from build123d import *

# Parameters (mm, degrees)
SKETCH2_R           = 49.2125
BOSS_EXTRUDE1_DEPTH = 50.8
SKETCH3_R           = 9.525
SKETCH4_R           = 49.2125
SKETCH4_R_2         = 9.525
BOSS_EXTRUDE2_DEPTH = 50.8


with BuildPart() as part:
    # Sketch1 → Revolve1 (revolve)
    with BuildSketch(Plane(origin=(0, 0, 0), x_dir=(0, 0, -1), z_dir=(1, 0, 0))):
        with BuildLine():
            Line((0, 0), (-304.8, 0))
            add(Edge.make_bspline(
                [(-304.8, 0), (-304.382425601, 0.143168366), (-303.540765888, 0.430899345), (-301.740901659, 1.044224359), (-299.788343499, 1.703616117), (-297.798910734, 2.370622283), (-295.782175929, 3.041960911), (-293.777683441, 3.704074038), (-291.768115862, 4.362899187), (-289.746498304, 5.020634276), (-287.712339913, 5.677355174), (-268.688556224, 11.771202945), (-231.321588698, 22.614032917), (-177.061866436, 35.203944952), (-118.24504839, 44.082248155), (-74.116427434, 48.134305599), (-47.14784979, 49.654737541), (-36.353282187, 50.114030962), (-28.794561554, 50.366026549), (-23.934493272, 50.49822726), (-20.694154368, 50.573944325), (-17.741054824, 50.63389122), (-15.603916609, 50.671594447), (-13.478042738, 50.704275318), (-11.363951605, 50.732021274), (-9.516855824, 50.752830907), (-7.391927552, 50.771857001), (-5.292027124, 50.786126656), (-3.234867855, 50.7956398), (-1.330315082, 50.799207238), (-0.441435733, 50.800000002), (0, 50.800000002)],
                knots=[0.082835744, 0.082835744, 0.082835744, 0.082835744, 0.082835744, 0.088524103, 0.094212462, 0.099900821, 0.10558918, 0.111277539, 0.116965898, 0.122654257, 0.128342616, 0.134156146, 0.139969677, 0.337629697, 0.546916774, 0.732949735, 0.779457974, 0.814339154, 0.837593273, 0.849220333, 0.860847393, 0.866660923, 0.872474453, 0.88100699, 0.88385117, 0.889539528, 0.895227886, 0.900916244, 0.906604603, 0.912292961, 0.917981319, 0.917981319, 0.917981319, 0.917981319, 0.917981319], degree=4))
            Line((0, 50.800000002), (0, 0))
        make_face()
    revolve(axis=Axis((0, 0, 0), (0, 0, 1)))

    # Sketch2 → Boss-Extrude1 (add)
    with BuildSketch(Plane(origin=(0, 0, 0), x_dir=(-1, 0, 0), z_dir=(0, 0, -1))):
        with Locations(Location((0, 0, 0), (0, 0, 90))):
            Circle(SKETCH2_R)
    extrude(amount=BOSS_EXTRUDE1_DEPTH)

    # Sketch3 → Cut-Revolve3 (revolve, cut)
    with BuildSketch(Plane(origin=(0, 0, -50.8), x_dir=(-1, 0, 0), z_dir=(0, 0, -1)), mode=Mode.PRIVATE) as cut_revolve3_sk:
        with Locations((-25.4, 0)):
            Circle(SKETCH3_R)
    revolve(cut_revolve3_sk.sketch.rotate(Axis((0, 0, -50.8), (0, 1, 0)), 270), axis=Axis((0, 0, -50.8), (0, 1, 0)), mode=Mode.SUBTRACT)

    # Sketch4 → Boss-Extrude2 (add)
    with BuildSketch(Plane(origin=(0, 0, -50.8), x_dir=(-1, 0, 0), z_dir=(0, 0, -1))):
        with Locations(Location((0, 0, 0), (0, 0, 90))):
            Circle(SKETCH4_R)
        with Locations(Location((-25.4, 0, 0), (0, 0, 180))):
            Circle(SKETCH4_R_2, mode=Mode.SUBTRACT)
        with Locations(Location((25.4, 0, 0), (0, 0, 270))):
            Circle(SKETCH4_R_2, mode=Mode.SUBTRACT)
    extrude(amount=BOSS_EXTRUDE2_DEPTH)


solid = part.part
The model under review builds one solid part; all positions refer to its coordinate system, in mm. Round coordinates to 2 decimals unless told otherwise and drop trailing zeros. Answer as a JSON object with one key per item and string values.
1. The part is to be moulded in two halves that separate along Y. For faces 1 (the face through (48.794, -6.406, -50.089)), 2 (the face through (-16.1, 2.06, -75.84)), 3 (the face through (1, -1, -101.6)), say which applies: pulls with the +Y half, pulls with the -Y half, needs draft (parallel to the pull), parting line crosses it, or undercut.
Results found:
{"face 1": "parting line crosses it", "face 2": "undercut", "face 3": "needs draft"}
2. To check wall thickness, follow line 1 along Y through (x, z) = (25, -66); line 2 along Y through (x, z) = (25.4, -78) (3 decimals); line 3 along Y through (x, z) = (5.5, 88). State the ranges of each line that lie inside material, in increasing order.
Results found:
{"line 1": "y = -42.39 to -9.52, 9.52 to 42.39", "line 2": "y = -42.151 to -9.525, 9.525 to 42.151", "line 3": "y = -46.35 to 46.35"}
3. Clearance check with flat-ended pins moving along their axes: pin 1 (8 mm diameter, centred on x = 13, z = 255.5, fed in from +Y); pin 2 (5 mm diameter, centred on y = 18, z = 94.5, fed in from +X); pin 3 (3 mm diameter, centred on y = 27.5, z = -38.5, fed in from -X). State where each tip first meets the part, or that it passes through.
Results found:
{"pin 1": "stops at y = 12.82", "pin 2": "stops at x = 43.39", "pin 3": "stops at x = -41.78"}
